Autodesk Fusion 360 part; units mm, degrees
sketch "Sketch1" plane through (0, 0, 0) normal (0, 0, 1) x (1, 0, 0) in component "bottom"
  line L0 (150, 110) -> (-150, 110)
  line L1 (-150, 110) -> (-150, -110)
  line L2 (-150, -110) -> (150, -110)
  line L3 (150, -110) -> (150, 110)
  line L4 (150, 110) -> (-150, -110) construction
  line L5 (-150, 110) -> (150, -110) construction
  dimension "d1" = 300
  dimension "d2" = 220
extrude "Extrude1" add sketch "Sketch1" along normal blind 70 in component "bottom"
sketch "Sketch2" plane through (150, 0, 0) normal (1, 0, 0) x (0, 1, 0) in component "bottom"
  line L0 (-110, 0) -> (110, 0)
  line L1 (110, 0) -> (110, 70)
  line L2 (110, 70) -> (-110, 70)
  line L3 (-110, 70) -> (-110, 0)
  line L4 (-12.5, 47.5) -> (12.5, 47.5)
  line L5 (12.5, 47.5) -> (12.5, 22.5)
  line L6 (12.5, 22.5) -> (-12.5, 22.5)
  line L7 (-12.5, 22.5) -> (-12.5, 47.5)
  line L8 (-12.5, 47.5) -> (12.5, 22.5) construction
  line L9 (12.5, 47.5) -> (-12.5, 22.5) construction
  line L10 (3.9, 31.1) -> (-3.9, 31.1)
  line L11 (-3.9, 31.1) -> (-3.9, 38.9)
  line L12 (-3.9, 38.9) -> (3.9, 38.9)
  line L13 (3.9, 38.9) -> (3.9, 31.1)
  point P0 (0, 35)
  dimension "d5" = 25
  dimension "d6" = 25
  dimension "d7" = 8.6
extrude "Extrude2" cut sketch "Sketch2" against normal blind 1.6 contours L10 L11 L12 L13 in component "bottom"
sketch "Sketch3" plane through (0, 0, 70) normal (0, 0, 1) x (-1, 0, 0) in component "bottom"
  line L0 (-150, 110) -> (-150, -110)
  line L1 (-150, -110) -> (150, -110)
  line L2 (150, -110) -> (150, 110)
  line L3 (150, 110) -> (-150, 110)
  line L4 (135, 95) -> (-135, 95)
  line L5 (-135, 95) -> (-135, -95)
  line L6 (-135, -95) -> (135, -95)
  line L7 (135, -95) -> (135, 95)
  dimension "d10" = -15
extrude "Extrude3" cut sketch "Sketch3" against normal up to surface (55 mm away) contours L4 L5 L6 L7 in component "bottom"
component "bottom" placed x (1, 0, 0) y (0, 1, 0) z (0, 0, 1) at (0, 0, 0)
component "top" placed x (1, 0, 0) y (0, 1, 0) z (0, 0, 1) at (0, 0, 0)
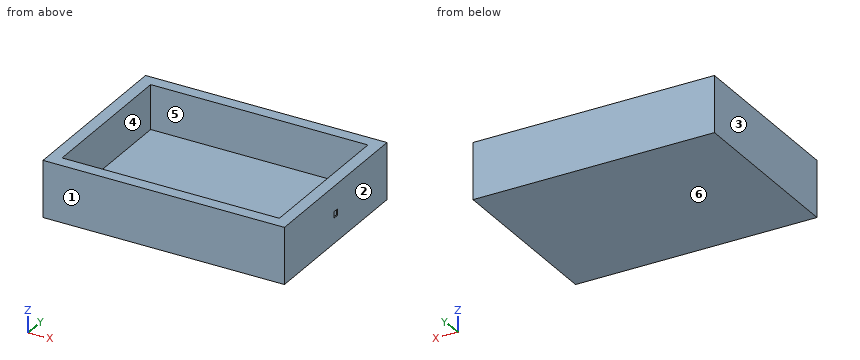
Build history of the part. All positions in model axes, mm. Face numbers are marked on the shaded views. A direction names the side the tool comes from. Coordinates: 2 decimals unless noted, no trailing zeros. Write each loop counter-clockwise with the first axis right and the second up, starting at its lowest first coordinate (ties: lowest second). Pieces come first, ordered by that corner, then holes.
(1) Drill centre lines: line 1 (X direction, y = -88, z = 42.5); line 2 (Y direction, x = -132.5, z = 24); line 3 (Z direction, x = -85, y = -6). Where is each one in solid material? Low to high.
(2) Cut at C-C on y = -67. List the corners of the cut face in (x, z).
(3) Mould opens along X. For the marked faces 1, 2, 3 and 4 say: pulls with the +X half, pulls with the -X half, needs draft (parallel to the pull), parting line crosses it, or undercut.
(4) Cut at B-B on z = 53. List the corners of the cut face in (x, y).
(5) Cut at A-A on x = -63. List the corners of the cut face in (y, z).
(6) 3-axis set-ups, long thin cutter, end or side, ignore diameter. For the marked faces 5 and 6: which of +Z, -Z, +X, -X, +Y, -Y reach the whole face in a straight line?
(7) Pin check, flat tip, straight feed: pin 1 Ø4 at (y, z) = (-0.5, 36.5) entering from +X. Stop position of the tip, or through.
Working result:
1. line 1: x = -150 to -135, 135 to 150
1. line 2: y = -110 to -95, 95 to 110
1. line 3: z = 0 to 15
2. outline: (-150, 0) - (150, 0) - (150, 70) - (135, 70) - (135, 15) - (-135, 15) - (-135, 70) - (-150, 70) - close
3. face 1: needs draft
3. face 2: pulls with the +X half
3. face 3: pulls with the -X half
3. face 4: undercut
4. outline: (-150, -110) - (150, -110) - (150, 110) - (-150, 110) - close; hole (-135, -95) - (135, -95) - (135, 95) - (-135, 95) - close
5. outline: (-110, 0) - (110, 0) - (110, 70) - (95, 70) - (95, 15) - (-95, 15) - (-95, 70) - (-110, 70) - close
6. face 5: +Z
6. face 6: -Z, +X, -X, +Y, -Y
7. pin 1: stops at x = 148.4
